For this review, take the finished solid that the model builds, in its own axes (mm). A direction names the side the tool comes from. Round coordinates to 2 decimals unless told otherwise and drop trailing zeros. Loops run counter-clockwise (first coordinate to the right, second up) from the corner with the lowest first, then second, coordinate; pieces in that order, holes last.
1. To check wall thickness, follow line 1 along Y through (x, z) = (5, -4.5); line 2 along Z through (x, y) = (15, 16.1); line 3 along Z through (x, y) = (1.75, 14). State the ranges of each line that lie inside material, in increasing order.
2. Draft analysis for pull direction Z (two halves, no side actions). For faces 3 (the flat face through (15, 17, -33)), 4 (the cylindrical face through (15.914, 16.972, -16.567)), 5 (the flat face through (15, -19, -15)), 6 (the cylindrical face through (15.914, -17.028, -16.567)), state which applies: released by +Z, released by -Z, zero draft, split by the parting line, or undercut.
3. Tool access review of faces 1 (the flat face through (15, 19, -15)), 2 (the flat face through (18, -4, -3)): name each direction out of +Z, -Z, +X, -X, +Y, -Y from which nothing blocks a thin tool from reaching the whole face with its end or side.
4. Consider section D-D on z = -1.5. State the section outline as (x, y) points, then the cut area to 3 significant figures.
5. Consider section C-C on y = 0. State the section outline as (x, z) points.
6. Clearance check with flat-ended pins moving along their axes: pin 1 Ø15 at (x, y) = (12.5, -4.5) entering from -Z; pin 2 Ø8 at (y, z) = (-12, -22.5) entering from -X. State where each tip first meets the part, or that it passes through.
7. Consider section B-B on x = 15. State the section outline as (y, z) points, then the cut area to 3 significant figures.
8. Consider section A-A on z = -24.5. State the section outline as (x, y) points.
from build123d import *

# Parameters (mm, degrees)
SKETCH2_W           = 6
SKETCH2_H           = 30
BOSS_EXTRUDE1_DEPTH = 30
SKETCH4_R           = 4
CUT_EXTRUDE2_DEPTH  = 30
SKETCH5_R           = 1.7
CUT_EXTRUDE3_DEPTH  = 39


with BuildPart() as part:
    # Sketch2 → Boss-Extrude1 (new body)
    with BuildSketch(Plane(origin=(0, 0, 0), x_dir=(0, 0, -1), z_dir=(1, 0, 0))):
        Rectangle(SKETCH2_W, SKETCH2_H)
        Polygon((-3, 19), (-3, 15), (3, 15), (33, 15), (33, 19), align=None)
        Polygon((3, -15), (-3, -15), (-3, -19), (33, -19), (33, -15), align=None)
    extrude(amount=BOSS_EXTRUDE1_DEPTH)

    # Sketch4 → Cut-Extrude2 (cut)
    with BuildSketch(Plane.XY.offset(3)):
        with Locations((15, 0)):
            Circle(SKETCH4_R)
    extrude(amount=-CUT_EXTRUDE2_DEPTH, mode=Mode.SUBTRACT)

    # Sketch5 → Cut-Extrude3 (cut, through all)
    with BuildSketch(Plane.XZ.offset(19)):
        with Locations((15, -18)):
            Circle(SKETCH5_R)
    extrude(amount=-CUT_EXTRUDE3_DEPTH, mode=Mode.SUBTRACT)


solid = part.part
Resolved:
1. line 1: y = -19 to -15, 15 to 19
1. line 2: z = -33 to -19.7, -16.3 to 3
1. line 3: z = -3 to 3
2. face 3: released by -Z
2. face 4: undercut
2. face 5: zero draft
2. face 6: undercut
3. face 1: +Z, -Z, +X, -X, +Y
3. face 2: -Z, +X, -X
4. outline: (0, -19) - (30, -19) - (30, 19) - (0, 19) - close; hole circle Ø8 at (15, 0)
4. area: 1,090 mm2
5. outline: (0, -3) - (11, -3) - (11, 3) - (0, 3) - close; (19, -3) - (30, -3) - (30, 3) - (19, 3) - close
6. pin 1: stops at z = -3
6. pin 2: stops at x = 0
7. outline: (-19, -33) - (-15, -33) - (-15, -19.7) - (-19, -19.7) - close; (-19, -16.3) - (-15, -16.3) - (-15, -3) - (-4, -3) - (-4, 3) - (-19, 3) - close; (4, -3) - (15, -3) - (15, -16.3) - (19, -16.3) - (19, 3) - (4, 3) - close; (15, -33) - (19, -33) - (19, -19.7) - (15, -19.7) - close
7. area: 393 mm2
8. outline: (0, -19) - (30, -19) - (30, -15) - (0, -15) - close; (0, 15) - (30, 15) - (30, 19) - (0, 19) - close
